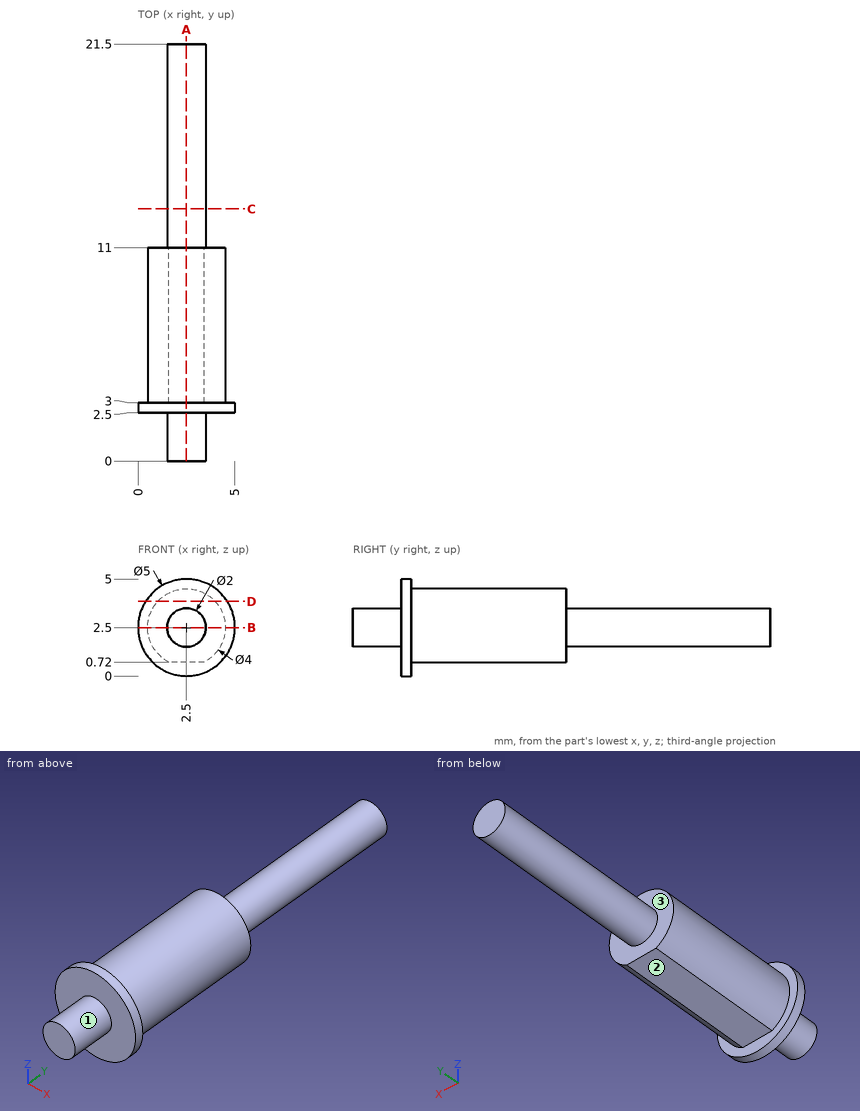
Input: dimensioned drawing with shaded views. Units: mm. Origin: part minimum x, y, z. A direction names the side the tool comes from. Round coordinates to 2 decimals unless told otherwise and drop trailing zeros. Order: outer loops, then holes, each group sorted by start corner. A loop starts at its lowest first (then second) coordinate and runs counter-clockwise, first axis right, second up. Notation, with made-up numbers: (47.25, -36) - (69.25, -36) arc R12 cw to (69.25, -17) - close; hole circle Ø8 at (15.5, -28). An arc over 180 degrees is marked (long way). Answer as a JSON object with one key per item and string values. Group by question number.
(1) Reachability of the marked faces 1, 2 and 3 from +Z, -Z, +X, -X, +Y, -Y: full face, straight path, thin tool, end or side. Return the list, or none.
(2) Cut plane A-A (x = 2.5). Return loops of the section in (y, z), then the cut area to 3 significant figures.
(3) Cut plane B-B (z = 2.5). Return loops of the section in (x, y).
(4) Material intervals for probe 1 along Y at (x, z) = (3.15, 3.7); probe 2 along Y at (x, z) = (4.3, 3.8); probe 3 along Z at (x, y) = (2.4, 6), sorted ascending. Write a range as from..to.
(5) Pin query (flat end, axial travel): P1, Ø1, axis at x = 1.5, y = 5.5, coming from the -Z side; P2, Ø3, axis at y = 9, z = 3, coming from the -X side; P3, Ø2, axis at y = 16, z = 3.5, coming from the +X side. Return the tip coordinate at first contact, or that it passes through.
(6) Cut plane C-C (y = 13). Return loops of the section in (x, z), then the cut area to 3 significant figures.
(7) Cut plane D-D (z = 3.85). Return loops of the section in (x, y), then the cut area to 3 significant figures.
Here are the results:
{
 "1": {"face 1": "-Y", "face 2": "-Z, +X, -X, +Y", "face 3": "+Y"},
 "2": {"outline": "(0, 1.5) - (2.5, 1.5) - (2.5, 0) - (3, 0) - (3, 0.72) - (11, 0.72) - (11, 1.5) - (21.5, 1.5) - (21.5, 3.5) - (11, 3.5) - (11, 4.5) - (3, 4.5) - (3, 5) - (2.5, 5) - (2.5, 3.5) - (0, 3.5) - close", "area": "58.7 mm^2"},
 "3": {"outline": "(0, 2.5) - (1.5, 2.5) - (1.5, 0) - (3.5, 0) - (3.5, 2.5) - (5, 2.5) - (5, 3) - (4.5, 3) - (4.5, 11) - (3.5, 11) - (3.5, 21.5) - (1.5, 21.5) - (1.5, 11) - (0.5, 11) - (0.5, 3) - (0, 3) - close"},
 "4": {"probe 1": "y = 2.5..11", "probe 2": "y = 2.5..3", "probe 3": "z = 0.72..4.5"},
 "5": {"P1": "stops at z = 0.72", "P2": "stops at x = 0.5", "P3": "stops at x = 3.5"},
 "6": {"outline": "circle Ø2 at (2.5, 2.5)", "area": "3.14 mm^2"},
 "7": {"outline": "(0.4, 2.5) - (4.6, 2.5) - (4.6, 3) - (3.98, 3) - (3.98, 11) - (1.02, 11) - (1.02, 3) - (0.4, 3) - close", "area": "25.7 mm^2"}
}
